from build123d import *

# Parameters (mm, degrees)
BOSS_EXTRUDE1_DEPTH = 4
SKETCH2_R           = 3
CUT_EXTRUDE1_DEPTH  = 33.264456547
SKETCH3_R           = 3
CUT_EXTRUDE2_DEPTH  = 33.264456547


with BuildPart() as part:
    # Sketch1 → Boss-Extrude1 (new, symmetric)
    with BuildSketch(Plane(origin=(0, 0, 0), x_dir=(1, 0, 0), z_dir=(0, 1, 0))):
        Polygon((-4, 19.8125), (4, 19.8125), (4, 21.4), (-4, 21.4), (-21.4, 21.4), (-21.4, 4), (-21.4, -4), (-19.8125, -4), (-19.8125, 4), (-19.8125, 19.8125), align=None)
    extrude(amount=BOSS_EXTRUDE1_DEPTH, both=True)

    # Sketch2 → Cut-Extrude1 (cut, through all)
    with BuildSketch(Plane(origin=(-19.8125, 0, 0), x_dir=(0, 0, -1), z_dir=(1, 0, 0))):
        Circle(SKETCH2_R)
    extrude(amount=-CUT_EXTRUDE1_DEPTH, mode=Mode.SUBTRACT)

    # Sketch3 → Cut-Extrude2 (cut, through all)
    with BuildSketch(Plane.XY.offset(-19.8125)):
        Circle(SKETCH3_R)
    extrude(amount=-CUT_EXTRUDE2_DEPTH, mode=Mode.SUBTRACT)


solid = part.part
Could you check a few things on this model? Use its own coordinates, in mm. A direction names the side the tool comes from. Coordinates: 2 decimals unless noted, no trailing zeros. Write each loop counter-clockwise with the first axis right and the second up, starting at its lowest first coordinate (ties: lowest second). Pieces come first, ordered by that corner, then holes. Notation, with made-up numbers: (45.5, 31) - (101.5, 31) arc R13 ccw to (101.5, 37) - close; hole circle Ø7 at (-36.5, 57). An arc over 180 degrees is marked (long way). Put each result on its own line as item: value. Start each with the question number.
Q1. Which directions (+Z, -Z, +X, -X, +Y, -Y) give clear straight access to the entire face, cutting with the end or side of a thin tool? Please do faces 1 (the flat face through (-11, 0, -21.4)), 2 (the flat face through (-19.812, 0, -10)).
Q2. I want a section at A-A on z = 0. Write out the boundary of the cut face in (x, y), plus the area to 4 significant figures.
Q3. I'm going to push flat-ended pins straight in: P1, Ø5, axis at x = -15.5, z = -2.5, coming from the +Y side; P2, Ø1, axis at y = 2, z = -7.5, coming from the +X side; P3, Ø4, axis at x = -8, y = 0.5, coming from the +Z side. Where does each tip first touch, or does it pass through?
Q4. I want a section at B-B on y = 0. Write out the boundary of the cut face in (x, z), plus the area to 3 significant figures.
Q5. Please list where these lines run through material, in increasing order: L1, parallel to Y at x = 0, z = -20.15; L2, parallel to Z at x = -19.5, y = -0.5.
Q6. I want a section at D-D on x = -16.75. Write out the boundary of the cut face in (y, z).
Q7. I want a section at C-C on x = 0. Write out the boundary of the cut face in (y, z), plus the area to 4 significant figures.
Q8. Thinking about a two-plate mould opening in X: for faces 3 (the flat face through (-20, -4, -14)), 4 (the flat face through (-21.4, 0, -12)), 5 (the cylindrical face through (-3, 0, -21)), 6 (the flat face through (4, 0, -21)), which applies, pulls with the +X half, pulls with the -X half, needs draft (parallel to the pull), parting line crosses it, or undercut?
Checks:
1. face 1: -Z, +X, -X, +Y, -Y
1. face 2: +Z, +X, +Y, -Y
2. outline: (-21.4, -4) - (-19.81, -4) - (-19.81, -3) - (-21.4, -3) - close; (-21.4, 3) - (-19.81, 3) - (-19.81, 4) - (-21.4, 4) - close
2. area: 3.175 mm²
3. P1: through
3. P2: x = -19.81
3. P3: z = -19.81
4. outline: (-21.4, -21.4) - (-3, -21.4) - (-3, -19.81) - (-19.81, -19.81) - (-19.81, -3) - (-21.4, -3) - close; (-21.4, 3) - (-19.81, 3) - (-19.81, 4) - (-21.4, 4) - close; (3, -21.4) - (4, -21.4) - (4, -19.81) - (3, -19.81) - close
4. area: 59.1 mm²
5. L1: -4 to -3, 3 to 4
5. L2: -21.4 to -19.81
6. outline: (-4, -21.4) - (4, -21.4) - (4, -19.81) - (-4, -19.81) - close
7. outline: (-4, -21.4) - (-3, -21.4) - (-3, -19.81) - (-4, -19.81) - close; (3, -21.4) - (4, -21.4) - (4, -19.81) - (3, -19.81) - close
7. area: 3.175 mm²
8. face 3: needs draft
8. face 4: pulls with the -X half
8. face 5: undercut
8. face 6: pulls with the +X half
